Verification items for the finished model (mm, model axes). A direction names the side the tool comes from. Give positions to 0.01 mm unless a question says otherwise; leave off trailing zeros. Loops run counter-clockwise (first coordinate to the right, second up) from the corner with the lowest first, then second, coordinate; pieces in that order, holes last. Notation, with made-up numbers: (38, 61) -> (93, 61) arc R12 ccw to (93, 84) -> close; hole circle Ø8 at (-27, 49). An arc over 180 degrees is marked (long way). Answer in a Markdown table with one row per item. Add a question column.
Q1. Material ranges on probe 1 along X at (y, z) = (6.25, 364); probe 2 along Z at (x, y) = (-468, 5.75); probe 3 along Z at (x, y) = (-194, 0.5), recorded low to high.
Q2. Release check for a two-part mould opening along Z. For faces 3 (the face through (-145.945, 4.93, 650.901)), 4 (the face through (-29.95, 4.93, 547.96)), 5 (the face through (-406, 0, 17)) record: pulls with the +Z half, pulls with the -Z half, needs draft (parallel to the pull), parting line crosses it, or undercut.
Q3. Section check C-C on y = 5.5. Enter the section's corners in (x, z).
Q4. Section check B-B on z = 489. Enter the section's corners in (x, y).
Q5. Gauge pin test, flat ends, axial feed: P1, Ø6, axis at y = 7.5, z = 640.5, coming from the -X side; P2, Ø1, axis at y = 6.5, z = 656, coming from the -X side. Record the tip position at first contact, or that the pin passes through.
Q6. Section check A-A on x = -366.5. Enter the section's corners in (y, z), and give its area (3 significant figures).
Q7. Set-up check for faces 1 (the face through (-406, 10, 17)), 2 (the face through (-749.744, 4.93, 532.545)): record each of +Z, -Z, +X, -X, +Y, -Y from which the full face is reachable in a straight line by a thin tool's end or side.
Autodesk Inventor part; units mm, degrees
ref_plane "YZ Plane" through (0, 0, 0) normal (1, 0, 0) x (0, 1, 0)
ref_plane "XZ Plane" through (0, 0, 0) normal (0, 1, 0) x (-1, 0, 0)
ref_plane "XY Plane" through (0, 0, 0) normal (0, 0, 1) x (1, 0, 0)
sketch "Skizze2" plane through (0, 0, 0) normal (0, 1, 0) x (-1, 0, 0)
  line L0 (326.749, 800) -> (176.0567, 737.5812)
  line L1 (176.0567, 737.5812) -> (60.7218, 622.2463)
  line L2 (60.7218, 622.2463) -> (-1.697, 471.5541)
  line L3 (-1.697, 471.5541) -> (-1.697, 0)
  line L4 (-1.697, 0) -> (0, 0)
  line L5 (0, 0) -> (816.6061, 0)
  line L6 (816.6061, 0) -> (818.303, 0)
  line L7 (818.303, 0) -> (818.303, 471.5541)
  line L8 (818.303, 471.5541) -> (755.8842, 622.2463)
  line L9 (755.8842, 622.2463) -> (640.5494, 737.5812)
  line L10 (640.5494, 737.5812) -> (489.8571, 800)
  line L11 (489.8571, 800) -> (326.749, 800)
  line L12 (617.8912, 76.3291) -> (481.9006, 20)
  line L13 (481.9006, 20) -> (334.7055, 20)
  line L14 (334.7055, 20) -> (198.7149, 76.3291)
  line L15 (198.7149, 76.3291) -> (94.6322, 180.4118)
  line L16 (94.6322, 180.4118) -> (38.303, 316.4024)
  line L17 (38.303, 316.4024) -> (38.303, 463.5976)
  line L18 (38.303, 463.5976) -> (94.6322, 599.5882)
  line L19 (94.6322, 599.5882) -> (198.7149, 703.6709)
  line L20 (198.7149, 703.6709) -> (334.7055, 760)
  line L21 (334.7055, 760) -> (481.9006, 760)
  line L22 (481.9006, 760) -> (617.8912, 703.6709)
  line L23 (617.8912, 703.6709) -> (721.9739, 599.5882)
  line L24 (721.9739, 599.5882) -> (778.303, 463.5976)
  line L25 (778.303, 463.5976) -> (778.303, 316.4024)
  line L26 (778.303, 316.4024) -> (721.9739, 180.4118)
  line L27 (721.9739, 180.4118) -> (617.8912, 76.3291)
  point P0 (481.9006, 20)
  dimension "d89" = 157.5
  dimension "d90" = 22.5
  dimension "d91" = 135
  dimension "d92" = 90
  dimension "d93" = 90
  dimension "d94" = 40
  dimension "d95" = 780
  dimension "d96" = 820
  dimension "d97" = 800
  dimension "d98" = 760
  dimension "d99" = 20
  dimension "d100" = 40
  dimension "d101" = 780
  dimension "d102" = 740
  dimension "d103" = 780
  dimension "d104" = 40
  dimension "d105" = 780
  dimension "d106" = 740
  dimension "d107" = 780
  dimension "d108" = 40
  dimension "d109" = 780
  dimension "d110" = 740
  dimension "d111" = 780
  dimension "d112" = 818.303
  dimension "d113" = 0
  dimension "d114" = 936.4693
  dimension "d115" = 597.9763
  dimension "d116" = 974.4855
  dimension "d117" = 382.9422
  dimension "d118" = 926.5638
  dimension "d119" = 165.9378
  dimension "d120" = 0
  dimension "d121" = 0
  dimension "d122" = 0
  dimension "d123" = 471.5541
  dimension "d124" = 0
  dimension "d125" = 0
  dimension "d126" = 1.697
  dimension "d127" = 1.697
  dimension "d128" = 40
  dimension "d129" = 463.5976
  dimension "d130" = 40
  dimension "d131" = 316.4024
  dimension "d132" = 62.4188
  dimension "d133" = 62.4188
  dimension "d134" = 96.3291
  dimension "d135" = 96.3291
  dimension "d136" = 96.3291
  dimension "d137" = 96.3291
  dimension "d138" = 177.7537
  dimension "d139" = 177.7537
  dimension "d140" = 200.4118
  dimension "d141" = 200.4118
  dimension "d142" = 200.4118
  dimension "d143" = 200.4118
  dimension "d144" = 328.4459
  dimension "d145" = 328.4459
  dimension "d146" = 336.4024
  dimension "d147" = 336.4024
  dimension "d148" = 336.4024
  dimension "d149" = 336.4024
  dimension "d150" = 483.5976
  dimension "d151" = 483.5976
  dimension "d152" = 483.5976
extrude "Extrusion1" add sketch "Skizze2" along normal blind 10
properties part number "Hauptplatte"
Taken from the geometry:
| question | item | result |
|---|---|---|
| 1 | probe 1 | x = -818.3 to -778.3, -38.3 to 1.7 |
| 1 | probe 2 | z = 0 to 20, 760 to 800 |
| 1 | probe 3 | z = 0 to 81.04, 698.96 to 745.01 |
| 2 | face 3 | undercut |
| 2 | face 4 | pulls with the +Z half |
| 2 | face 5 | needs draft |
| 3 | outline | (-818.3, 0) -> (1.7, 0) -> (1.7, 471.55) -> (-60.72, 622.25) -> (-176.06, 737.58) -> (-326.75, 800) -> (-489.86, 800) -> (-640.55, 737.58) -> (-755.88, 622.25) -> (-818.3, 471.55) -> close; hole (-778.3, 316.4) -> (-721.97, 180.41) -> (-617.89, 76.33) -> (-481.9, 20) -> (-334.71, 20) -> (-198.71, 76.33) -> (-94.63, 180.41) -> (-38.3, 316.4) -> (-38.3, 463.6) -> (-94.63, 599.59) -> (-198.71, 703.67) -> (-334.71, 760) -> (-481.9, 760) -> (-617.89, 703.67) -> (-721.97, 599.59) -> (-778.3, 463.6) -> close |
| 4 | outline | (-811.08, 0) -> (-767.78, 0) -> (-767.78, 10) -> (-811.08, 10) -> close; (-48.83, 0) -> (-5.53, 0) -> (-5.53, 10) -> (-48.83, 10) -> close |
| 5 | P1 | stops at x = -740.63 |
| 5 | P2 | stops at x = -722.63 |
| 6 | outline | (0, 0) -> (10, 0) -> (10, 20) -> (0, 20) -> close; (0, 760) -> (10, 760) -> (10, 800) -> (0, 800) -> close |
| 6 | area | 600 mm² |
| 7 | face 1 | +Z, -Z, +X, -X, +Y |
| 7 | face 2 | +Y, -Y |
